Check sheet for the drawn part. Datum: minimum x, y, z corner. Units: mm. Round coordinates to 2 decimals unless told otherwise and drop trailing zeros. Order: outer loops, then holes, each group sorted by start corner. A loop starts at its lowest first (then second) coordinate and runs counter-clockwise, first axis right, second up. Notation, with made-up numbers: M 76.25,-2.75 L 103.25,-2.75 A24 cw 103.25,9.25 Z; hole C -23.75,68 d5. An arc over 180 degrees is marked long. Use one line per item in the form item = value. Start each with the question number.
Item 1: Thickness scan on probe 1 along Y at (x, z) = (227.5, 1.9); probe 2 along X at (y, z) = (3, 2.8); probe 3 along X at (y, z) = (43, 2.85). Record the ranges inside material, lowest first. Write a range as [from, to].
Item 2: Go/stop test with a flat-tipped pin: pin 1 Ø2.5 at (x, y) = (2.5, 2.5) entering from -Z. Record where the tip stops, or that it passes through.
Item 3: Cross-section at A-A on x = 119.5. Enter the section's corners in (y, z).
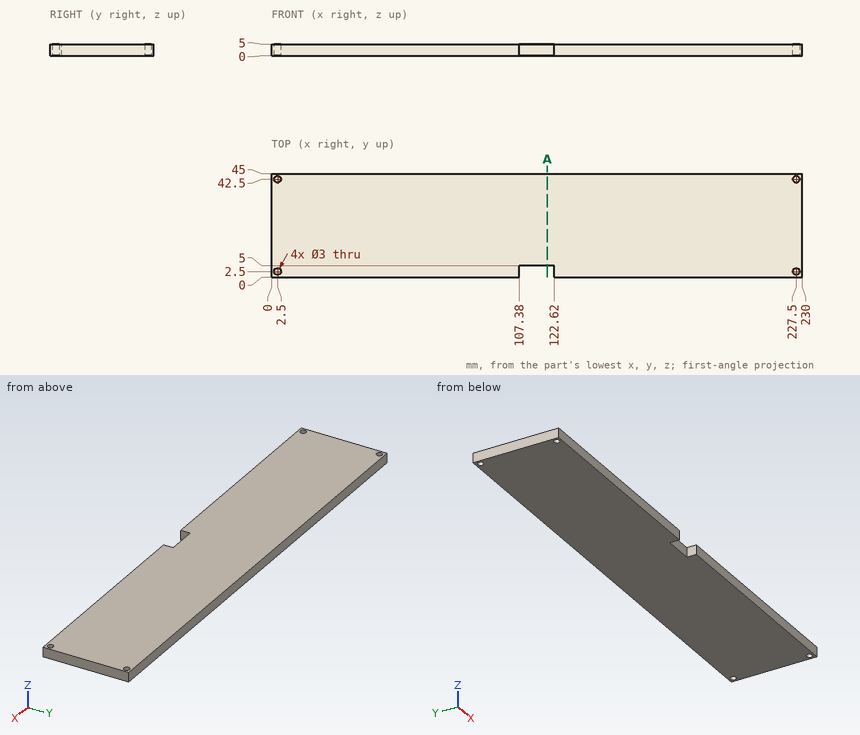
Output values:
q1.probe_1 = [0, 1], [4, 41], [44, 45]
q1.probe_2 = [0, 1.09], [3.91, 107.38], [122.62, 226.09], [228.91, 230]
q1.probe_3 = [0, 1.09], [3.91, 226.09], [228.91, 230]
q2.pin_1 = through
q3.outline = M 5,0 L 45,0 L 45,5 L 5,5 Z
